from build123d import *

# Parameters (mm, degrees)
ESQUISSE1_R                  = 5.549450549
ESQUISSE1_W                  = 8
ESQUISSE1_H                  = 94.34065934
ESQUISSE1_W_2                = 70
ESQUISSE1_H_2                = 70
BOSS_EXTRU_1_DEPTH           = 5
ESQUISSE4_R                  = 2
ENL_V_MAT_EXTRU_5_DEPTH      = 350
ESQUISSE9_W                  = 8
ESQUISSE9_H                  = 94.34065934
BOSS_EXTRU_2_DEPTH           = 5
BOSS_EXTRU_4_DEPTH           = 5
ESQUISSE11_W                 = 7
ESQUISSE11_H                 = 7
BOSS_EXTRU_6_DEPTH           = 340
ENL_V_MAT_EXTRU_6_DEPTH      = 10
ENL_V_MAT_EXTRU_6_DEPTH_BACK = 10
ESQUISSE12_R                 = 2
ESQUISSE14_R                 = 1
BOSS_EXTRU_8_DEPTH           = 10
SYM_TRIE1_START              = -10
SYM_TRIE1_OUTLINE_R          = 1
SYM_TRIE1_DEPTH              = 40
ESQUISSE15_W                 = 5
ESQUISSE15_H                 = 10.313810077
ENL_V_MAT_EXTRU_7_DEPTH      = 5
ESQUISSE17_W                 = 250
ESQUISSE17_H                 = 313.215569532
BOSS_EXTRU_9_DEPTH           = 3
ESQUISSE18_W                 = 190
ESQUISSE18_H                 = 270
ENL_V_MAT_EXTRU_8_DEPTH      = 24


# Read off the part's stored shape, not the designer's step: Symétrie1
with BuildPart() as part:
    # Esquisse1 → Boss.-Extru.1 (new body)
    with BuildSketch(Plane(origin=(0, 0, 0), x_dir=(1, 0, 0), z_dir=(0, 1, 0))):
        Polygon((-125, 166.483516484), (125, 166.483516484), (163.846153846, 122.087912088), (163.846153846, -122.087912088), (125, -166.483516484), (-125, -166.483516484), (-163.846153846, -122.087912088), (-163.846153846, 122.087912088), align=None)
        with Locations(Location((-133.846153846, 130.967032967, 0), (0, 0, 270))):
            Circle(ESQUISSE1_R, mode=Mode.SUBTRACT)
        with Locations(Location((-133.846153846, -130.967032967, 0), (0, 0, 90))):
            Circle(ESQUISSE1_R, mode=Mode.SUBTRACT)
        with Locations(Location((133.846153846, -130.967032967, 0), (0, 0, 270))):
            Circle(ESQUISSE1_R, mode=Mode.SUBTRACT)
        with Locations(Location((133.846153846, 130.967032967, 0), (0, 0, 90))):
            Circle(ESQUISSE1_R, mode=Mode.SUBTRACT)
        with Locations((-144, 0)):
            Rectangle(ESQUISSE1_W, ESQUISSE1_H, mode=Mode.SUBTRACT)
        with Locations((87.5, 0)):
            Rectangle(ESQUISSE1_W_2, ESQUISSE1_H_2, mode=Mode.SUBTRACT)
        with Locations((-87.5, 0)):
            Rectangle(ESQUISSE1_W_2, ESQUISSE1_H_2, mode=Mode.SUBTRACT)
        with Locations((144, 0)):
            Rectangle(ESQUISSE1_W, ESQUISSE1_H, mode=Mode.SUBTRACT)
    extrude(amount=BOSS_EXTRU_1_DEPTH)

    # Esquisse4 → Enlèv. mat.-Extru.5 (cut)
    with BuildSketch(Plane(origin=(0, 5, 0), x_dir=(1, 0, 0), z_dir=(0, 1, 0))):
        with Locations(Location((-157.846153846, 67, 0), (0, 0, 270))):
            Circle(ESQUISSE4_R)
        with Locations(Location((157.846153846, 67, 0), (0, 0, 90))):
            Circle(ESQUISSE4_R)
        with Locations(Location((-157.846153846, -67, 0), (0, 0, 90))):
            Circle(ESQUISSE4_R)
        with Locations(Location((157.846153846, -67, 0), (0, 0, 270))):
            Circle(ESQUISSE4_R)
    extrude(amount=-ENL_V_MAT_EXTRU_5_DEPTH, mode=Mode.SUBTRACT)

    # Esquisse9 → Boss.-Extru.2 (add)
    with BuildSketch(Plane(origin=(0, 5, 0), x_dir=(1, 0, 0), z_dir=(0, 1, 0))):
        with Locations((-144, 0)):
            Rectangle(ESQUISSE9_W, ESQUISSE9_H)
        with Locations((144, 0)):
            Rectangle(ESQUISSE9_W, ESQUISSE9_H)
    extrude(amount=-BOSS_EXTRU_2_DEPTH)

    # Esquisse10 → Boss.-Extru.4 (add)
    with BuildSketch(Plane(origin=(0, 5, 0), x_dir=(1, 0, 0), z_dir=(0, 1, 0))):
        Polygon((-125, 206.483516484), (-144.423076923, 144.285714286), (144.423076923, 144.285714286), (125, 206.483516484), align=None)
        Polygon((125, -206.483516484), (144.423076923, -144.285714286), (-144.423076923, -144.285714286), (-125, -206.483516484), align=None)
    extrude(amount=-BOSS_EXTRU_4_DEPTH)

    # Esquisse11 → Boss.-Extru.6 (add)
    with BuildSketch(Plane(origin=(0, 5, 0), x_dir=(1, 0, 0), z_dir=(0, 1, 0))):
        with Locations((121.5, -153.107784766)):
            Rectangle(ESQUISSE11_W, ESQUISSE11_H)
        with Locations((-121.5, -153.107784766)):
            Rectangle(ESQUISSE11_W, ESQUISSE11_H)
        with Locations((121.5, 153.107784766)):
            Rectangle(ESQUISSE11_W, ESQUISSE11_H)
        with Locations((-121.5, 153.107784766)):
            Rectangle(ESQUISSE11_W, ESQUISSE11_H)
    extrude(amount=BOSS_EXTRU_6_DEPTH)

    # Esquisse12 → Enlèv. mat.-Extru.6 (cut, two sides: drawn at the far end of the back side and taken through both)
    with BuildSketch(Plane(origin=(0, 5, 0), x_dir=(1, 0, 0), z_dir=(0, 1, 0)).offset(-ENL_V_MAT_EXTRU_6_DEPTH_BACK)):
        with Locations(Location((-55, 186.483516484, 0), (0, 0, 90))):
            Circle(ESQUISSE12_R)
        with Locations(Location((55, 186.483516484, 0), (0, 0, 90))):
            Circle(ESQUISSE12_R)
        with Locations(Location((55, -186.483516484, 0), (0, 0, 90))):
            Circle(ESQUISSE12_R)
        with Locations(Location((-55, -186.483516484, 0), (0, 0, 90))):
            Circle(ESQUISSE12_R)
    extrude(amount=ENL_V_MAT_EXTRU_6_DEPTH + ENL_V_MAT_EXTRU_6_DEPTH_BACK, mode=Mode.SUBTRACT)

    # Esquisse14 → Boss.-Extru.8 (add, symmetric)
    with BuildSketch(Plane(origin=(0, 0, 0), x_dir=(0, 0, -1), z_dir=(1, 0, 0))):
        with BuildLine():
            Line((206.483516484, 5), (211.463094512, 5))
            ThreePointArc((211.463094512, 5), (213.963094512, 2.5), (211.463094512, 0))
            Line((211.463094512, 0), (206.483516484, 0))
            Line((206.483516484, 0), (206.483516484, 5))
        make_face()
        with Locations((208.973305498, 2.5)):
            Circle(ESQUISSE14_R, mode=Mode.SUBTRACT)
    extrude(amount=BOSS_EXTRU_8_DEPTH, both=True)

    # Symétrie1 outline → Symétrie1 (add)
    # profile 1 of 2: a face of its own
    with BuildSketch(Plane.YZ.offset(SYM_TRIE1_START)):
        with BuildLine():
            Line((0, -206.483516484), (0, -211.463094512))
            ThreePointArc((0, -211.463094512), (2.5, -213.963094512), (5, -211.463094512))
            Line((5, -211.463094512), (5, -206.483516484))
            Line((5, -206.483516484), (0, -206.483516484))
        make_face()
        with Locations((2.5, -208.973305498)):
            Circle(SYM_TRIE1_OUTLINE_R, mode=Mode.SUBTRACT)
    # profile 2 of 2: a face of its own
    with BuildSketch(Plane.YZ.offset(SYM_TRIE1_START)):
        with BuildLine():
            Line((0, 211.463094512), (0, 206.483516484))
            Line((0, 206.483516484), (5, 206.483516484))
            Line((5, 206.483516484), (5, 211.463094512))
            ThreePointArc((5, 211.463094512), (2.5, 213.963094512), (0, 211.463094512))
        make_face()
        with Locations((2.5, 208.973305498)):
            Circle(SYM_TRIE1_OUTLINE_R, mode=Mode.SUBTRACT)
    extrude(amount=SYM_TRIE1_DEPTH)

    # Esquisse15 → Enlèv. mat.-Extru.7 (cut)
    with BuildSketch(Plane(origin=(0, 5, 0), x_dir=(1, 0, 0), z_dir=(0, 1, 0))):
        with Locations((-7.5, 211.640421522)):
            Rectangle(ESQUISSE15_W, ESQUISSE15_H)
        with Locations((27.5, 211.640421522)):
            Rectangle(ESQUISSE15_W, ESQUISSE15_H)
        with Locations((27.5, -211.640421522)):
            Rectangle(ESQUISSE15_W, ESQUISSE15_H)
        with Locations((-7.5, -211.640421522)):
            Rectangle(ESQUISSE15_W, ESQUISSE15_H)
    extrude(amount=-ENL_V_MAT_EXTRU_7_DEPTH, mode=Mode.SUBTRACT)

    # Esquisse17 → Boss.-Extru.9 (add)
    with BuildSketch(Plane(origin=(0, 345, 0), x_dir=(1, 0, 0), z_dir=(0, 1, 0))):
        Rectangle(ESQUISSE17_W, ESQUISSE17_H)
    extrude(amount=-BOSS_EXTRU_9_DEPTH)

    # Esquisse18 → Enlèv. mat.-Extru.8 (cut)
    with BuildSketch(Plane(origin=(0, 345, 0), x_dir=(1, 0, 0), z_dir=(0, 1, 0))):
        Rectangle(ESQUISSE18_W, ESQUISSE18_H)
    extrude(amount=-ENL_V_MAT_EXTRU_8_DEPTH, mode=Mode.SUBTRACT)


solid = part.part
The listing builds one solid part. Answer for the finished solid, in the listing's coordinates (mm). A direction names the side the tool comes from. Coordinates: 2 decimals unless noted, no trailing zeros. Write each loop counter-clockwise with the first axis right and the second up, starting at its lowest first coordinate (ties: lowest second). Pieces come first, ordered by that corner, then holes. Notation, with made-up numbers: (42.5, 33) - (53.5, 33) arc R24 cw to (53.5, 49) - close; hole circle Ø11 at (89.25, 60.25). An arc over 180 degrees is marked (long way). Put each result on its own line as item: value.
1. Find the intervals of material crossed by line 1 along X through (y, z) = (3.75, 67); line 2 along Z through (x, y) = (10.5, 2.5); line 3 along Y through (x, z) = (109, -80.5), in increasing order. Write a range as from..to.
Answer sheet:
line 1: x = -163.85..-159.85, -155.85..155.85, 159.85..163.85
line 2: z = -213.96..-209.97, -207.97..207.97, 209.97..213.96
line 3: y = 0..5, 342..345
2. Flat-ended cylindrical pins translate along their axes: pin 1 Ø3 at (x, z) = (55, 186.48) entering from -Y; pin 2 Ø2 at (x, y) = (121, 101.5) entering from -Z; pin 3 Ø5 at (x, z) = (-157.85, -67) entering from +Y; pin 4 Ø3.5 at (y, z) = (209.5, -153) entering from -X. Find the tip coordinate at first contact, or state that the pin passes through.
Answer sheet:
pin 1: passes through
pin 2: stops at z = -156.61
pin 3: stops at y = 5
pin 4: stops at x = -125
3. The part is cut by section C-C on x = -72.5. Give the vertices of the cut face in (y, z), plus the area to 3 significant figures.
Answer sheet:
outline: (0, -206.48) - (5, -206.48) - (5, -35) - (0, -35) - close; (0, 35) - (5, 35) - (5, 206.48) - (0, 206.48) - close; (342, -156.61) - (345, -156.61) - (345, -135) - (342, -135) - close; (342, 135) - (345, 135) - (345, 156.61) - (342, 156.61) - close
area: 1,840 mm^2
4. The part is cut by section D-D on z = 11.5. Give the vertices of the cut face in (x, y), plus the area to 3 significant figures.
Answer sheet:
outline: (-163.85, 0) - (-122.5, 0) - (-122.5, 5) - (-163.85, 5) - close; (-125, 342) - (-95, 342) - (-95, 345) - (-125, 345) - close; (-52.5, 0) - (52.5, 0) - (52.5, 5) - (-52.5, 5) - close; (95, 342) - (125, 342) - (125, 345) - (95, 345) - close; (122.5, 0) - (163.85, 0) - (163.85, 5) - (122.5, 5) - close
area: 1,120 mm^2
5. The part is cut by section B-B on z = -55. Give the vertices of the cut face in (x, y).
Answer sheet:
outline: (-163.85, 0) - (163.85, 0) - (163.85, 5) - (-163.85, 5) - close; (-125, 342) - (-95, 342) - (-95, 345) - (-125, 345) - close; (95, 342) - (125, 342) - (125, 345) - (95, 345) - close
6. A tool of negligible diameter and unlimited length cuts with its end or side. For faces 1 (the face through (-125, 174, -150)), 2 (the face through (-131.72, 2.46, 125.84)), 3 (the face through (-121, 174, -156.608)), 4 (the face through (125, 174, -150)), from which of +Z, -Z, +X, -X, +Y, -Y can it reach the whole face along a straight path? Write none if from no direction.
Answer sheet:
face 1: +Z, -Z, -X, +Y
face 2: +Y, -Y
face 3: -Z, +X, -X, +Y
face 4: +Z, -Z, +X, +Y
7. Determine the mould class of faces 5 (the face through (138.77, 2.46, -133.53)), 6 (the face through (134.576, 2.535, 175.82)), 7 (the face through (-154.3, 2.5, -133)), 8 (the face through (-121, 174, 156.608)) for opening direction X: pulls with the +X half, pulls with the -X half, needs draft (parallel to the pull), parting line crosses it, or undercut.
Answer sheet:
face 5: undercut
face 6: pulls with the +X half
face 7: pulls with the -X half
face 8: needs draft
8. The part is cut by section A-A on y = 23.5. Give the vertices of the cut face in (x, z), plus the area to 3 significant figures.
Answer sheet:
outline: (-125, -156.61) - (-118, -156.61) - (-118, -149.61) - (-125, -149.61) - close; (-125, 149.61) - (-118, 149.61) - (-118, 156.61) - (-125, 156.61) - close; (118, -156.61) - (125, -156.61) - (125, -149.61) - (118, -149.61) - close; (118, 149.61) - (125, 149.61) - (125, 156.61) - (118, 156.61) - close
area: 196 mm^2
